Geometry check sheet. Reference: the model listing, model coordinates, mm. Face numbers are marked on the shaded views. A direction names the side the tool comes from. Give positions to 0.01 mm unless a question says otherwise; leave off trailing zeros. Write each loop counter-clockwise with the first axis right and the second up, starting at its lowest first coordinate (ties: lowest second). Pieces come first, ordered by that corner, then holes. Notation, with made-up numbers: (58.25, 59.25) -> (93.25, 59.25) arc R7 ccw to (93.25, 67.25) -> close; hole circle Ø3 at (28.5, 2.5). An arc over 180 degrees is marked (long way). One line per item, written item: value.
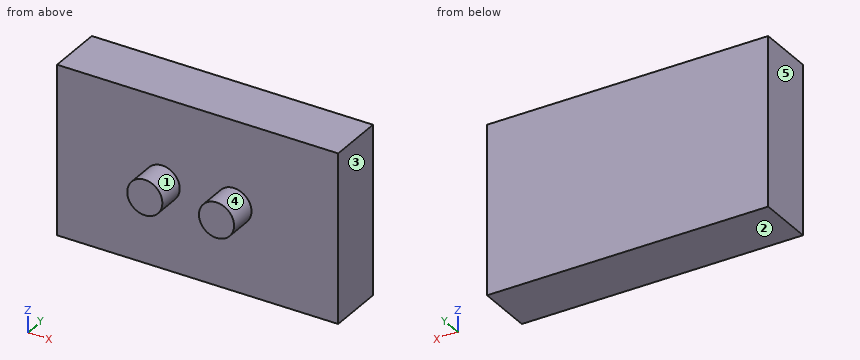
from build123d import *

# Parameters (mm, degrees)
F0_W     = 127
F0_H     = 76.2
F1_DEPTH = 25.4
F2_R     = 7.9375
F3_DEPTH = 12.7


with BuildPart() as f1:
    # F0 (on Front) → F1 (new body)
    with BuildSketch(Plane.XZ):
        Rectangle(F0_W, F0_H)
    extrude(amount=-F1_DEPTH)

    # F2 (on Front) → F3 (join)
    with BuildSketch(Plane.XZ):
        with Locations((-16.006199, 0)):
            Circle(F2_R)
        with Locations((16.378801, 0)):
            Circle(F2_R)
    extrude(amount=F3_DEPTH)


solid = f1.part
1) Depth check by flat-ended pin: pin 1 Ø6 at (x, z) = (31, 9.5) entering from -Y. Enter the tip coordinate at first touch or a pass-through.
Verdict:
pin 1: y = 0
2) Tool access check on the marked faces 4 and 5. Record the directions out of +Z, -Z, +X, -X, +Y, -Y that give a thin tool (end or side, any length) a straight path to the whole face; none if there is none.
Verdict:
face 4: -Y
face 5: +Z, -Z, -X, +Y, -Y
3) Mould release check, pull along X, two halves, no side actions. Record for the marked faces 1, 2 and 3: released by +X, released by -X, zero draft, split by the parting line, or undercut.
Verdict:
face 1: undercut
face 2: zero draft
face 3: released by +X
4) Scan lines: probe 1 along Y at (x, z) = (47, 3.5); probe 2 along Z at (x, y) = (23, -10); probe 3 along Z at (x, y) = (-14, -0.5). Record each from-to range of solid material in increasing order.
Verdict:
probe 1: 0 to 25.4
probe 2: -4.38 to 4.38
probe 3: -7.68 to 7.68
5) Sectioned sample at C-C on y = -4. Record the cut outline in (x, z) (1 decimal).
Verdict:
outline: circle Ø15.9 at (-16, 0); circle Ø15.9 at (16.4, 0)
6) Sectioned sample at D-D on x = 51. Record the cut outline in (y, z).
Verdict:
outline: (0, -38.1) -> (25.4, -38.1) -> (25.4, 38.1) -> (0, 38.1) -> close
7) Sectioned sample at A-A on z = 0. Record the cut outline in (x, y), plus the area to 3 significant figures.
Verdict:
outline: (-63.5, 0) -> (-23.94, 0) -> (-23.94, -12.7) -> (-8.07, -12.7) -> (-8.07, 0) -> (8.44, 0) -> (8.44, -12.7) -> (24.32, -12.7) -> (24.32, 0) -> (63.5, 0) -> (63.5, 25.4) -> (-63.5, 25.4) -> close
area: 3,630 mm^2
8) Sectioned sample at B-B on x = -22.5. Record the cut outline in (y, z).
Verdict:
outline: (-12.7, -4.56) -> (0, -4.56) -> (0, -38.1) -> (25.4, -38.1) -> (25.4, 38.1) -> (0, 38.1) -> (0, 4.56) -> (-12.7, 4.56) -> close
